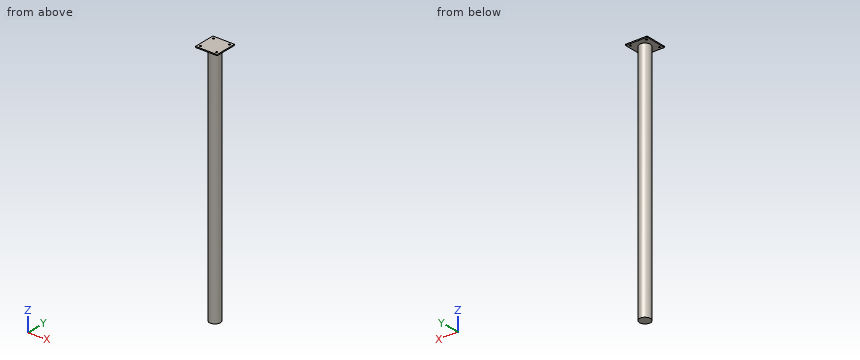
```python
from build123d import *

# Parameters (mm, degrees)
F0_R     = 16
F1_DEPTH = 700
F2_W     = 62
F2_H     = 62
F3_DEPTH = 3
F4_R     = 2.5
F5_DEPTH = 3


with BuildPart() as f1:
    # F0 (on Top) → F1 (new body)
    with BuildSketch(Plane.XY):
        Circle(F0_R)
    extrude(amount=-F1_DEPTH)

    # F2 (on Top) → F3 (join)
    with BuildSketch(Plane.XY):
        Rectangle(F2_W, F2_H)
    extrude(amount=-F3_DEPTH)

    # F4 (on Top) → F5 (cut, through all)
    with BuildSketch(Plane.XY):
        with Locations((-23, 23)):
            Circle(F4_R)
        with Locations((23, 23)):
            Circle(F4_R)
        with Locations((23, -23)):
            Circle(F4_R)
        with Locations((-23, -23)):
            Circle(F4_R)
    extrude(amount=-F5_DEPTH, mode=Mode.SUBTRACT)


solid = f1.part
```
Read the model definition and answer for the solid it produces. Units are mm, in the model's axes. Round coordinates to 2 decimals unless told otherwise and drop trailing zeros. Write each loop counter-clockwise with the first axis right and the second up, starting at its lowest first coordinate (ties: lowest second). Pieces come first, ordered by that corner, then holes. Notation, with made-up numbers: M 14.25,86 L 31.25,86 A25 ccw 31.25,113 Z; hole C 22,69.5 d5. An arc over 180 degrees is marked long. One line per item, written item: value.
Q1. Find section B-B on x = -3. Write down the section's boundary in (y, z), plus the area to 3 significant figures.
Data:
outline: M -31,-3 L -15.72,-3 L -15.72,-700 L 15.72,-700 L 15.72,-3 L 31,-3 L 31,0 L -31,0 Z
area: 22,100 mm2
Q2. Find section C-C on z = -284.5. Write down the section's boundary in (x, y), plus the area to 3 significant figures.
Data:
outline: C 0,0 d32
area: 804 mm2
Q3. Flat-ended cylindrical pins translate along their axes: pin 1 Ø10 at (y, z) = (-7, -555) entering from -X; pin 2 Ø8 at (x, y) = (-23, -23) entering from -Z; pin 3 Ø8 at (x, z) = (18.5, -454) entering from -Y. Find the tip coordinate at first contact, or state that the pin passes through.
Data:
pin 1: x = -15.87
pin 2: z = -3
pin 3: y = -6.76
Q4. Straight lines are drawn through the part: line 1 (Y direction, x = 23, z = -1.8); line 2 (Z direction, x = 12.5, y = -23); line 3 (Y direction, x = -2, z = -283.5). For each, find the intervals that lie inside material, in ascending order. Write a range as [from, to].
Data:
line 1: [-31, -25.5], [-20.5, 20.5], [25.5, 31]
line 2: [-3, 0]
line 3: [-15.87, 15.87]
Q5. Find section A-A on y = 0. Write down the section's boundary in (x, z).
Data:
outline: M -31,-3 L -16,-3 L -16,-700 L 16,-700 L 16,-3 L 31,-3 L 31,0 L -31,0 Z
